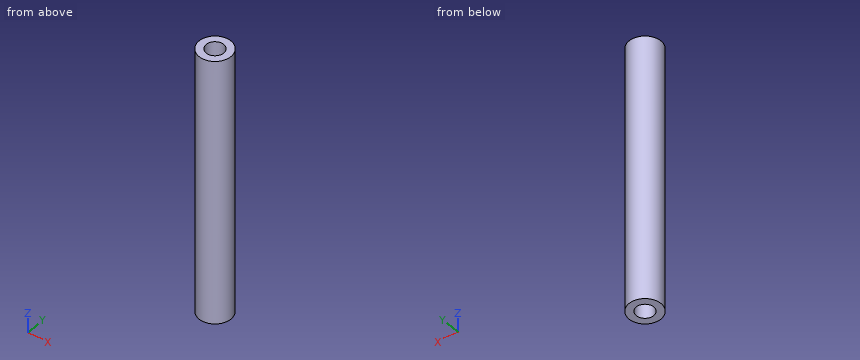
from build123d import *

# Parameters (mm, degrees)
SCHIZZO1_R                   = 2.985
ESTRUSIONE_ESTRUSIONE1_DEPTH = 24.91
SCHIZZO2_R                   = 1.6
TAGLIO_ESTRUSIONE1_DEPTH     = 50.998528478


with BuildPart() as part:
    # Schizzo1 → Estrusione-Estrusione1 (new, symmetric)
    with BuildSketch(Plane.XY):
        Circle(SCHIZZO1_R)
    extrude(amount=ESTRUSIONE_ESTRUSIONE1_DEPTH, both=True)

    # Schizzo2 → Taglio-Estrusione1 (cut, through all)
    with BuildSketch(Plane.XY.offset(24.91)):
        Circle(SCHIZZO2_R)
    extrude(amount=-TAGLIO_ESTRUSIONE1_DEPTH, mode=Mode.SUBTRACT)

    # Schizzo3 → Foro filettato M4x0.7-1 (revolve, cut)
    with BuildSketch(Plane(origin=(0, 0, 24.91), x_dir=(0, -1, 0), z_dir=(1, 0, 0))):
        Polygon((0, 0), (0, 12.991420021), (1.65, 12), (1.65, 0), align=None)
    foro_filettato_m4x0_7_1 = revolve(axis=Axis((0, 0, 31.26), (0, 0, -1)), mode=Mode.SUBTRACT)

    # Specchia1: Foro filettato M4x0.7-1 across plane
    add(foro_filettato_m4x0_7_1.mirror(Plane.XY), mode=Mode.SUBTRACT)


solid = part.part
CAD build for the part. Positions are in the model's coordinates, mm. Give positions to 0.01 mm unless a question says otherwise; leave off trailing zeros. Write each loop counter-clockwise with the first axis right and the second up, starting at its lowest first coordinate (ties: lowest second). Pieces come first, ordered by that corner, then holes. Notation, with made-up numbers: (-23.5, -6) - (-5.5, -6) arc R27 cw to (-5.5, 29) - close; hole circle Ø1 at (55, -4.75). An arc over 180 degrees is marked (long way). Answer as CSV lines item,"result".
Q1. Drill centre lines: line 1 (Y direction, x = -0.05, z = -22); line 2 (X direction, y = -0.5, z = -16.5); line 3 (Y direction, x = -0.75, z = 11). Where is each one in solid material? Low to high. Write a range as from..to.
Result set:
line 1,"-2.98..-1.65, 1.65..2.98"
line 2,"-2.94..-1.57, 1.57..2.94"
line 3,"-2.89..-1.41, 1.41..2.89"
Q2. Band-saw the part on C-C (z = -7). Give the cut face in (x, y) (3 decimals), and give its area (3 significant figures).
Result set:
outline,"circle Ø5.97 at (0, 0); hole circle Ø3.2 at (0, 0)"
area,"19.9 mm²"
Q3. Band-saw the part on D-D (z = -22). Give the cut face in (x, y) (3 decimals).
Result set:
outline,"circle Ø5.97 at (0, 0); hole circle Ø3.3 at (0, 0)"
Q4. Flat gauge pins, fed straight in: pin 1 Ø2 at (x, y) = (0, 0) entering from +Z; pin 2 Ø2 at (y, z) = (0.5, -17.5) entering from -X (3 decimals); pin 3 Ø3 at (x, z) = (-2, -11.5) entering from -Y; pin 4 Ø1 at (x, z) = (2, -15.5) entering from +Y. Where does each tip first touch, or does it go through?
Result set:
pin 1,"through"
pin 2,"x = -2.985"
pin 3,"y = -2.94"
pin 4,"y = 2.58"
Q5. Band-saw the part on A-A (y = 0). Give the cut face in (x, z) (3 decimals).
Result set:
outline,"(-2.985, -24.91) - (-1.65, -24.91) - (-1.65, -12.91) - (-1.6, -12.88) - (-1.6, 12.88) - (-1.65, 12.91) - (-1.65, 24.91) - (-2.985, 24.91) - close; (1.6, -12.88) - (1.65, -12.91) - (1.65, -24.91) - (2.985, -24.91) - (2.985, 24.91) - (1.65, 24.91) - (1.65, 12.91) - (1.6, 12.88) - close"
